The model under review builds one solid part; all positions refer to its coordinate system, in mm. A direction names the side the tool comes from. Round coordinates to 2 decimals unless told otherwise and drop trailing zeros. Write each loop counter-clockwise with the first axis right and the second up, starting at its lowest first coordinate (ties: lowest second). Pieces come first, ordered by that corner, then holes. Notation, with made-up numbers: (67.5, -23) -> (93.5, -23) arc R18 ccw to (93.5, -15) -> close; hole circle Ø2 at (74, 50.5). An arc over 180 degrees is marked (long way). Return JSON: item names as keys, results as strings. Group by question number.
1. Take a section at A-A, the plane y = 13.25. Write out the cut boundary in (x, z), then the cut area to 3 significant figures.
2. Clearance check with flat-ended pins moving along their axes: P1, Ø8, axis at x = -42.5, z = 2, coming from the +Y side; P2, Ø8, axis at x = -38.5, y = 4, coming from the -Z side; P3, Ø10, axis at x = -17, y = -1, coming from the -Z side; P4, Ø3, axis at x = -16, y = 2.5, coming from the -Z side. State where each tip first meets the part, or that it passes through.
3. Mouldability with a two-part tool opening along X and no side actions: class faces 1 (the flat face through (-43.244, 9.423, -2.986)), 2 (the cylindrical face through (52.5, -2.4, -7.8)), 3 (the cylindrical face through (-32.5, 0.1, 0.1)) as pulls with the +X half, pulls with the -X half, needs draft (parallel to the pull), parting line crosses it, or undercut.
4. Tool access review of faces 4 (the cylindrical face through (-49, 12, 0)), 5 (the flat face through (-41.536, 9, 0)), 6 (the flat face through (1, -5, -9)), 7 (the flat face through (1, 0, 5)): name each direction out of +Z, -Z, +X, -X, +Y, -Y from which nothing blocks a thin tool from reaching the whole face with its end or side.
5. Take a section at B-B, the plane y = 0. Write out the cut boundary in (x, z).
6. Take a section at D-D, the plane x = 44. Write out the cut boundary in (y, z).
7. For line 1 along Y through (x, z) = (42.5, -8); line 2 along X through (y, z) = (8.5, -12.5); line 3 along Z through (x, y) = (-36.5, 13), list the stretches that pass through material, from the lowest coordinate up. Write a range as from..to.
8. Take a section at C-C, the plane z = -11.5. Write out the cut boundary in (x, y).
from build123d import *

# Parameters (mm, degrees)
BOSS_EXTRUDE1_DEPTH     = 50
SKETCH2_R               = 12.5
CUT_EXTRUDE1_DEPTH      = 4
CUT_EXTRUDE3_DEPTH      = 54.677276384
CUT_EXTRUDE3_DEPTH_BACK = 54.677276384
SKETCH6_R               = 2
CUT_EXTRUDE4_DEPTH      = 4
SKETCH7_R               = 4
BOSS_EXTRUDE3_DEPTH     = 5


with BuildPart() as part:
    # Sketch1 → Boss-Extrude1 (new, symmetric)
    with BuildSketch(Plane(origin=(0, 0, 0), x_dir=(0, 0, -1), z_dir=(1, 0, 0))):
        Polygon((5, 5), (10, 10), (5, 15), (-5, 15), (-10, 10), (-5, 5), (-5, -5), (-12.5, -5), (-12.5, -8), (12.5, -8), (12.5, -5), (5, -5), align=None)
    extrude(amount=BOSS_EXTRUDE1_DEPTH, both=True)

    # Sketch2 → Cut-Extrude1 (cut, symmetric)
    with BuildSketch(Plane(origin=(0, 0, 0), x_dir=(1, 0, 0), z_dir=(0, 1, 0))):
        with Locations((-45, 0)):
            Circle(SKETCH2_R)
    extrude(amount=CUT_EXTRUDE1_DEPTH, both=True, mode=Mode.SUBTRACT)

    # Sketch4 → Cut-Extrude3 (cut, two sides: drawn at the far end of the back side and taken through both)
    with BuildSketch(Plane(origin=(0, 0, 0), x_dir=(1, 0, 0), z_dir=(0, 1, 0)).offset(-CUT_EXTRUDE3_DEPTH_BACK)):
        Polygon((-45, -4), (-41.535898385, -2), (-41.535898385, 2), (-45, 4), (-48.464101615, 2), (-48.464101615, -2), align=None)
    extrude(amount=CUT_EXTRUDE3_DEPTH + CUT_EXTRUDE3_DEPTH_BACK, mode=Mode.SUBTRACT)

    # Sketch6 → Cut-Extrude4 (cut)
    with BuildSketch(Plane.ZY.offset(50)):
        with Locations((0, 10)):
            Circle(SKETCH6_R)
    extrude(amount=-CUT_EXTRUDE4_DEPTH, mode=Mode.SUBTRACT)

    # Sketch7 → Boss-Extrude3 (add)
    with BuildSketch(Plane(origin=(50, 0, 0), x_dir=(0, 0, -1), z_dir=(1, 0, 0))):
        with BuildLine():
            Line((10, 10), (15.094664958, 7.034466496))
            ThreePointArc((15.094664958, 7.034466496), (19.020839401, -1.384245389), (12.5, -8))
            Line((12.5, -8), (-12.5, -8))
            ThreePointArc((-12.5, -8), (-19.020839401, -1.384245389), (-15.094664958, 7.034466496))
            Line((-15.094664958, 7.034466496), (-10, 10))
            Line((-10, 10), (-5, 15))
            Line((-5, 15), (5, 15))
            Line((5, 15), (10, 10))
        make_face()
        with Locations((11, 0)):
            Circle(SKETCH7_R, mode=Mode.SUBTRACT)
        with Locations(Location((-11, 0, 0), (0, 0, 180))):
            Circle(SKETCH7_R, mode=Mode.SUBTRACT)
    extrude(amount=BOSS_EXTRUDE3_DEPTH)


solid = part.part
Output:
{
 "1": {"outline": "(-50, -6.75) -> (55, -6.75) -> (55, 6.75) -> (-50, 6.75) -> close; hole (-48.46, -2) -> (-45, -4) -> (-41.54, -2) -> (-41.54, 2) -> (-45, 4) -> (-48.46, 2) -> close", "area": "1,380 mm^2"},
 "2": {"P1": "stops at y = 15", "P2": "stops at z = -8", "P3": "stops at z = -12.5", "P4": "stops at z = -5"},
 "3": {"face 1": "undercut", "face 2": "needs draft", "face 3": "pulls with the -X half"},
 "4": {"face 4": "-X", "face 5": "+Y, -Y", "face 6": "-Z, -X", "face 7": "+Z, -X"},
 "5": {"outline": "(-33.54, -5) -> (50, -5) -> (50, -7) -> (55, -7) -> (55, 7) -> (50, 7) -> (50, 5) -> (-33.54, 5) arc R12.5 cw to start; (50, -19.14) -> (55, -19.14) -> (55, -15) -> (50, -15) -> close; (50, 15) -> (55, 15) -> (55, 19.14) -> (50, 19.14) -> close"},
 "6": {"outline": "(-8, -12.5) -> (-5, -12.5) -> (-5, -5) -> (5, -5) -> (10, -10) -> (15, -5) -> (15, 5) -> (10, 10) -> (5, 5) -> (-5, 5) -> (-5, 12.5) -> (-8, 12.5) -> close"},
 "7": {"line 1": "y = -8..-5, 8..12", "line 2": "x = 50..55", "line 3": "z = -7..7"},
 "8": {"outline": "(-50, -8) -> (55, -8) -> (55, -3.97) -> (50, -3.97) -> (50, -5) -> (-50, -5) -> close; (50, 3.97) -> (55, 3.97) -> (55, 9.13) -> (50, 9.13) -> close"}
}
